```python
from build123d import *

# Parameters (mm, degrees)
F0_W     = 101.6
F0_H     = 50.8
F1_DEPTH = 76.2
F2_R     = 5.08
F3_T     = -2.54


# Not quite as in the source:
# - a shell that OpenCascade refuses in one call is made with other operations: the cavity is built on its own and cut out


with BuildPart() as f1:
    # F0 (on Front) → F1 (new body)
    with BuildSketch(Plane.XZ):
        with Locations((11.4285616755, 25.4)):
            Rectangle(F0_W, F0_H)
    extrude(amount=F1_DEPTH)

    # F2
    f2_edges = [f1.edges().sort_by_distance(p)[0] for p in [
        (-39.371438, -76.2, 25.4),
        (-39.371438, 0, 25.4),
        (11.428562, 0, 50.8),
        (62.228562, 0, 25.4),
    ]]
    fillet(f2_edges, radius=F2_R)

    # F3: a shell. OpenCascade refuses it in one call, so the cavity is built on its own and cut out:
    # the body offset inwards by the wall thickness, plus a prism from it out through each open face.
    f3_core = offset(f1.part, amount=F3_T, mode=Mode.PRIVATE)
    f3_exits = [f3_core.faces().sort_by_distance(p)[0] for p in [
        (12.698562, -73.66, 25.4),
    ]]
    add(f3_core, mode=Mode.SUBTRACT)
    extrude(f3_exits, amount=-F3_T, mode=Mode.SUBTRACT)


solid = f1.part
```
Can you work these out from the model? Positions are in its coordinate system, mm. A direction names the side the tool comes from. Coordinates: 2 decimals unless noted, no trailing zeros. Loops run counter-clockwise (first coordinate to the right, second up) from the corner with the lowest first, then second, coordinate; pieces in that order, holes last.
1) Imagine slicing it at C-C on z = 41. List the corners of the cut face in (x, y) for me, plus the area to 3 significant figures.
2) Imagine slicing it at A-A on y = -17. List the corners of the cut face in (x, z) for me, plus the area to 3 significant figures.
3) Imagine slicing it at B-B on x = 48. List the corners of the cut face in (y, z) for me.
4) I need wall thicknesses on probe 1 along X at (y, z) = (-62, 43); probe 2 along Z at (x, y) = (20.5, -37); probe 3 along Y at (x, z) = (-1, 23). Which ranges of each line are inside material? Lowest first, please.
5) Which directions (+Z, -Z, +X, -X, +Y, -Y) give clear straight access to the entire face, cutting with the end or side of a thin tool? Please do faces 1 (the flat face through (-36.831, -38, 25)), 2 (the cylindrical face through (58.96, -3.3, 25.72)), 3 (the flat face through (62.229, -40, 25)).
6) For pin 1 (1.5 mm diameter, centred on x = -4, z = 45, fed in from -Y), with a flat end and sliding along its axis, tell me the tip position at first contact or that it passes through.
7) Thinking about a two-plate mould opening in Y: for faces 4 (the cylindrical face through (60.78, -1.53, 25.76)), 5 (the cylindrical face through (-36.107, -3.304, 25.72)), 6 (the cylindrical face through (-37.923, -74.672, 25.756)), which applies, pulls with the +Y half, pulls with the -Y half, needs draft (parallel to the pull), parting line crosses it, or undercut?
Completed:
1. outline: (-39.37, -71.12) arc R5.08 ccw to (-34.29, -76.2) - (-34.29, -73.66) arc R2.54 cw to (-36.83, -71.12) - (-36.83, -5.08) arc R2.54 cw to (-34.29, -2.54) - (57.15, -2.54) arc R2.54 cw to (59.69, -5.08) - (59.69, -76.2) - (62.23, -76.2) - (62.23, -5.08) arc R5.08 ccw to (57.15, 0) - (-34.29, 0) arc R5.08 ccw to (-39.37, -5.08) - close
1. area: 626 mm2
2. outline: (-39.37, 0) - (62.23, 0) - (62.23, 50.8) - (-39.37, 50.8) - close; hole (-36.83, 2.54) - (59.69, 2.54) - (59.69, 48.26) - (-36.83, 48.26) - close
2. area: 748 mm2
3. outline: (-76.2, 0) - (0, 0) - (0, 45.72) arc R5.08 ccw to (-5.08, 50.8) - (-76.2, 50.8) - (-76.2, 48.26) - (-5.08, 48.26) arc R2.54 cw to (-2.54, 45.72) - (-2.54, 2.54) - (-76.2, 2.54) - close
4. probe 1: x = -39.37 to -36.83, 59.69 to 62.23
4. probe 2: z = 0 to 2.54, 48.26 to 50.8
4. probe 3: y = -2.54 to 0
5. face 1: none
5. face 2: -Y
5. face 3: +Z, -Z, +X, +Y, -Y
6. pin 1: stops at y = -2.54
7. face 4: pulls with the +Y half
7. face 5: undercut
7. face 6: pulls with the -Y half
